For this review, take the finished solid that the model builds, in its own axes (mm). Give positions to 0.01 mm unless a question says otherwise; leave off trailing zeros. Order: outer loops, then holes, each group sorted by start corner. A loop starts at its lowest first (then second) coordinate and runs counter-clockwise, first axis right, second up. Notation, with made-up numbers: (49, 46.5) -> (90, 46.5) arc R22 ccw to (90, 83.5) -> close; hole circle Ø4 at (53, -33). An arc over 180 degrees is marked (long way). One line per item, written item: value. Start each with the question number.
from build123d import *

# Parameters (mm, degrees)
F1_DEPTH = 69.85
F2_R     = 5.08
F3_R     = 6.35
F4_DEPTH = 19.051


with BuildPart() as f1:
    # F0 (on Top) → F1 (new body)
    with BuildSketch(Plane.XY):
        with BuildLine():
            Line((15.875, 9.525), (-15.875, 9.525))
            ThreePointArc((-15.875, 9.525), (-25.4, 0), (-15.875, -9.525))
            Line((-15.875, -9.525), (15.875, -9.525))
            ThreePointArc((15.875, -9.525), (25.4, 0), (15.875, 9.525))
        make_face()
    extrude(amount=F1_DEPTH)

    # F2
    f2_edges = [f1.edges().sort_by_distance(p)[0] for p in [
        (0, -9.525, 69.85),
        (25.4, 0, 69.85),
        (0, 9.525, 69.85),
        (-25.4, 0, 69.85),
        (0, -9.525, 0),
        (25.4, 0, 0),
        (0, 9.525, 0),
        (-25.4, 0, 0),
    ]]
    fillet(f2_edges, radius=F2_R)

    # F3 (on face) → F4 (cut, through all)
    with BuildSketch(Plane(origin=(0, 9.525, 0), x_dir=(-1, 0, 0), z_dir=(0, 1, 0))):
        with Locations((0, 50.8)):
            Circle(F3_R)
    extrude(amount=-F4_DEPTH, mode=Mode.SUBTRACT)


solid = f1.part
Q1. For line 1 along Z through (x, y) = (0, 2.5); line 2 along X through (y, z) = (-0.25, 29); line 3 along Z through (x, y) = (0, 5.25), list the stretches that pass through material, from the lowest coordinate up.
Q2. For pin 1 Ø2 at (x, z) = (-20, 60.5) entering from +Y; pin 2 Ø4 at (y, z) = (7, 55.5) entering from +X, all flat-tipped, find the tip position at first contact; note any pin that passes through.
Q3. Take a section at C-C (x = -13). State the section outline as (y, z) points (3 decimals), and give its area (3 significant figures).
Q4. Take a section at A-A (x = 0). State the section outline as (y, z) points (3 decimals), and give its area (3 significant figures).
Q5. Mouldability with a two-part tool opening along Z and no side actions: class faces 1 (the flat face through (0, 0, 0)), 2 (the cylindrical face through (25.398, -0.209, 34.507)), 3 (the cylindrical face through (0.8, 0.1, 57.1)), 4 (the cylindrical face through (0.2, -8.1, 68.3)) as pulls with the +Z half, pulls with the -Z half, needs draft (parallel to the pull), parting line crosses it, or undercut.
Q6. Take a section at B-B (z = 50.8). State the section outline as (x, y) points (3 decimals), and give its area (3 significant figures).
Q7. Take a section at D-D (x = -5.5). State the section outline as (y, z) points (3 decimals), and give its area (3 significant figures).
Answers below:
1. line 1: z = 0 to 44.45, 57.15 to 69.85
1. line 2: x = -25.4 to 25.4
1. line 3: z = 0.06 to 44.45, 57.15 to 69.79
2. pin 1: stops at y = 9
2. pin 2: stops at x = 23.98
3. outline: (-9.525, 5.08) arc R5.08 ccw to (-4.445, 0) -> (4.445, 0) arc R5.08 ccw to (9.525, 5.08) -> (9.525, 64.77) arc R5.08 ccw to (4.445, 69.85) -> (-4.445, 69.85) arc R5.08 ccw to (-9.525, 64.77) -> close
3. area: 1,310 mm²
4. outline: (-9.525, 5.08) arc R5.08 ccw to (-4.445, 0) -> (4.445, 0) arc R5.08 ccw to (9.525, 5.08) -> (9.525, 44.45) -> (-9.525, 44.45) -> close; (-9.525, 57.15) -> (9.525, 57.15) -> (9.525, 64.77) arc R5.08 ccw to (4.445, 69.85) -> (-4.445, 69.85) arc R5.08 ccw to (-9.525, 64.77) -> close
4. area: 1,070 mm²
5. face 1: pulls with the -Z half
5. face 2: needs draft
5. face 3: undercut
5. face 4: pulls with the +Z half
6. outline: (-15.875, -9.525) -> (-6.35, -9.525) -> (-6.35, 9.525) -> (-15.875, 9.525) arc R9.525 ccw to start; (6.35, -9.525) -> (15.875, -9.525) arc R9.525 ccw to (15.875, 9.525) -> (6.35, 9.525) -> close
6. area: 648 mm²
7. outline: (-9.525, 5.08) arc R5.08 ccw to (-4.445, 0) -> (4.445, 0) arc R5.08 ccw to (9.525, 5.08) -> (9.525, 47.626) -> (-9.525, 47.626) -> close; (-9.525, 53.974) -> (9.525, 53.974) -> (9.525, 64.77) arc R5.08 ccw to (4.445, 69.85) -> (-4.445, 69.85) arc R5.08 ccw to (-9.525, 64.77) -> close
7. area: 1,190 mm²
